Answer from the drawing. Dimensions are ordinates in mm from the lowest x, y and z of the part. A direction names the side the tool comes from. Give positions to 0.01 mm unless a question says otherwise; leave off trailing zeros. Order: outer loops, then holes, each group sorted by start corner. A loop starts at its lowest first (then second) coordinate and runs counter-clockwise, first axis right, second up. Notation, with made-up numbers: (-1.75, -18.75) - (40.25, -18.75) arc R8 ccw to (40.25, -7.75) - close; hole circle Ø2 at (-19.5, 77). An arc over 180 degrees is marked (long way). Write each question's results on one line, items separated by ' | '.
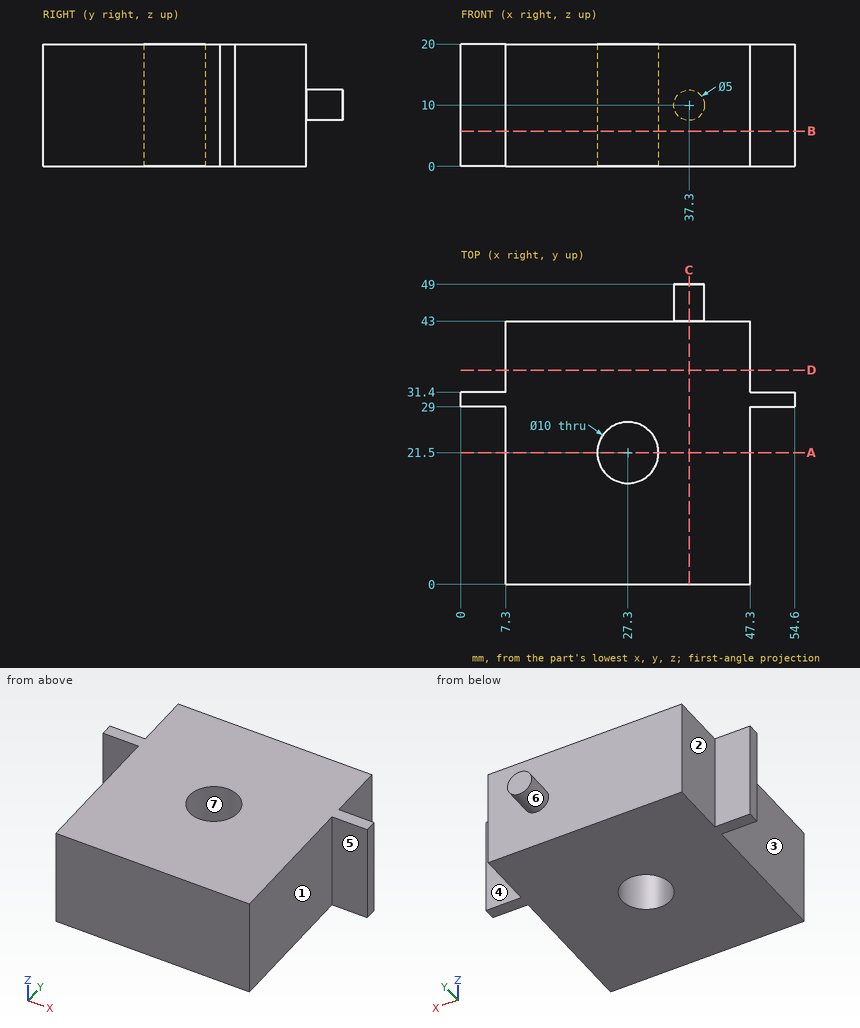
(1) Consider probe 1 along X at (y, z) = (37, 5.25); probe 2 along Y at (x, z) = (34, 15.25); probe 3 along X at (y, z) = (24.5, 6). Determine where each line is inside the solid, lowest interval first. Write a range as [from, to].
Conclusion:
probe 1: [7.3, 47.3] | probe 2: [0, 43] | probe 3: [7.3, 23.3], [31.3, 47.3]
(2) Section D-D (y = 35) is taken. Give the vertices of the cut face in (x, z), plus the area to 3 significant figures.
Conclusion:
outline: (7.3, 0) - (47.3, 0) - (47.3, 20) - (7.3, 20) - close | area: 800 mm^2
(3) The mould has two halves that part along Y. Classify the marked faces 5, 6 and 7: pulls with the +Y half, pulls with the -Y half, needs draft (parallel to the pull), parting line crosses it, or undercut.
Conclusion:
face 5: pulls with the -Y half | face 6: needs draft | face 7: undercut
(4) Section A-A (y = 21.5) is taken. Give the vertices of the cut face in (x, z).
Conclusion:
outline: (7.3, 0) - (22.3, 0) - (22.3, 20) - (7.3, 20) - close; (32.3, 0) - (47.3, 0) - (47.3, 20) - (32.3, 20) - close
(5) For the marked faces 1, 2, 3 and 4, determine the directions among +Z, -Z, +X, -X, +Y, -Y from which every point of the face is accessible in a straight line to the end or side of a thin tool.
Conclusion:
face 1: +Z, -Z, +X, -Y | face 2: +Z, -Z, -X, +Y | face 3: +Z, -Z, -X, -Y | face 4: +Z, -Z, +X, +Y
(6) Section C-C (x = 37.3) is taken. Give the vertices of the cut face in (y, z), plus the area to 3 significant figures.
Conclusion:
outline: (0, 0) - (43, 0) - (43, 7.5) - (49, 7.5) - (49, 12.5) - (43, 12.5) - (43, 20) - (0, 20) - close | area: 890 mm^2
(7) Each of these flat-tipped pins is pushed along its axis until it touches: pin 1 (6 mm diameter, centred on y = 36, z = 12, fed in from +X); pin 2 (10 mm diameter, centred on x = 28, z = 18, fed in from +Y); pin 3 (3.5 mm diameter, centred on x = 52.5, z = 6.5, fed in from -Y); pin 4 (8 mm diameter, centred on x = 27.3, y = 21.5, fed in from +Z). Where does it stop, or does it pass through?
Conclusion:
pin 1: x = 47.3 | pin 2: y = 43 | pin 3: y = 29 | pin 4: through
(8) Section B-B (z = 5.75) is taken. Give the vertices of the cut face in (x, y).
Conclusion:
outline: (0, 29) - (7.3, 29) - (7.3, 0) - (47.3, 0) - (47.3, 29) - (54.6, 29) - (54.6, 31.4) - (47.3, 31.4) - (47.3, 43) - (7.3, 43) - (7.3, 31.4) - (0, 31.4) - close; hole circle Ø10 at (27.3, 21.5)
